```python
from build123d import *

# Parameters (mm, degrees)
BOSS_EXTRUDE2_DEPTH = 5
SKETCH2_R           = 2.5
CUT_EXTRUDE1_DEPTH  = 5
SKETCH3_R           = 7
SKETCH3_R_2         = 1
CUT_EXTRUDE2_DEPTH  = 90.644870735
SKETCH4_R           = 1.5
CUT_EXTRUDE3_DEPTH  = 90.644870735
SKETCH5_R           = 1
CUT_EXTRUDE4_DEPTH  = 90.644870735


with BuildPart() as part:
    # Sketch1 → Boss-Extrude2 (new body)
    with BuildSketch(Plane(origin=(0, 0, 0), x_dir=(-1, 0, 0), z_dir=(0, 1, 0))):
        Polygon((-72.491053579, -52.5), (42.508946421, -52.5), (28.132122167, -13), (-65.526137841, -13), align=None)
    extrude(amount=BOSS_EXTRUDE2_DEPTH)

    # Sketch2 → Cut-Extrude1 (cut)
    with BuildSketch(Plane(origin=(0, 5, 0), x_dir=(-1, 0, 0), z_dir=(0, 1, 0))):
        with Locations(Location((28.227466353, -42.5, 0), (0, 0, 90))):
            Circle(SKETCH2_R)
        with Locations(Location((0, -22.5, 0), (0, 0, 90))):
            Circle(SKETCH2_R)
        with Locations(Location((-60.573517653, -42.5, 0), (0, 0, 90))):
            Circle(SKETCH2_R)
    extrude(amount=-CUT_EXTRUDE1_DEPTH, mode=Mode.SUBTRACT)

    # Sketch3 → Cut-Extrude2 (cut, through all)
    with BuildSketch(Plane(origin=(0, 5, 0), x_dir=(1, 0, 0), z_dir=(0, 1, 0))):
        with Locations(Location((29.491053579, 32, 0), (0, 0, 270))):
            Circle(SKETCH3_R)
        with Locations(Location((20.491053579, 32, 0), (0, 0, 270))):
            Circle(SKETCH3_R_2)
        with Locations(Location((29.491053579, 41, 0), (0, 0, 270))):
            Circle(SKETCH3_R_2)
        with Locations(Location((38.491053579, 32, 0), (0, 0, 270))):
            Circle(SKETCH3_R_2)
        with Locations(Location((29.491053579, 23, 0), (0, 0, 270))):
            Circle(SKETCH3_R_2)
    extrude(amount=-CUT_EXTRUDE2_DEPTH, mode=Mode.SUBTRACT)

    # Sketch4 → Cut-Extrude3 (cut, through all)
    with BuildSketch(Plane.XZ):
        with Locations(Location((-24.785336663, -15.5, 0), (0, 0, 270))):
            Circle(SKETCH4_R)
        with Locations(Location((10.214663337, -15.5, 0), (0, 0, 270))):
            Circle(SKETCH4_R)
        with Locations(Location((45.214663337, -15.5, 0), (0, 0, 270))):
            Circle(SKETCH4_R)
        with Locations(Location((63.861406816, -17.95576741, 0), (0, 0, 270))):
            Circle(SKETCH4_R)
        with Locations(Location((66.466129481, -32.727883705, 0), (0, 0, 270))):
            Circle(SKETCH4_R)
        with Locations(Location((69.070852146, -47.5, 0), (0, 0, 270))):
            Circle(SKETCH4_R)
    extrude(amount=-CUT_EXTRUDE3_DEPTH, mode=Mode.SUBTRACT)

    # Sketch5 → Cut-Extrude4 (cut, through all)
    with BuildSketch(Plane(origin=(0, 5, 0), x_dir=(-1, 0, 0), z_dir=(0, 1, 0))):
        with Locations(Location((37.295727555, -46.948212084, 0), (0, 0, 90))):
            Circle(SKETCH5_R)
    extrude(amount=-CUT_EXTRUDE4_DEPTH, mode=Mode.SUBTRACT)


solid = part.part
```
Here's how the part is built. I have some questions about the finished solid (model axes, mm). Give positions to 0.01 mm unless a question says otherwise; leave off trailing zeros. Write each loop counter-clockwise with the first axis right and the second up, starting at its lowest first coordinate (ties: lowest second). Pieces come first, ordered by that corner, then holes. Notation, with made-up numbers: M 35.5,-17.5 L 53.5,-17.5 A25 cw 53.5,10.5 Z; hole C -5.5,14.5 d10. An arc over 180 degrees is marked long. Put each result on its own line as item: value. Start each with the question number.
Item 1: I need wall thicknesses on L1, parallel to Z at x = 29.5, y = 3.3; L2, parallel to Z at x = 10, y = 0.3; L3, parallel to X at y = 4.5, z = -16. Which ranges of each line are inside material? Lowest first, please. Write a range as from..to.
Item 2: If we section it at C-C, the plane y = 2.95: Count the separate pieces of the cut face and the enclosed holes in it, then the cut area to 3 significant figures.
Item 3: Thinking about a two-plate mould opening in Z: for faces 1 (the flat face through (16, 0, -32)), 2 (the cylindrical face through (68.16, 2.46, -46.31)), 3 (the flat face through (16, 2, -52.5)), which applies, +Z half, -Z half, draft (parallel to the pull), parting line (faces both ways), or undercut?
Item 4: Will this pin go through, and if not, where does the flat tip stop? pin 1 (8.5 mm diameter, centred on x = 29.49, z = -32, fed in from -Y).
Item 5: If we section it at A-A, the plane z = -38: Write out the boundary of the cut face in (x, y), then the cut area to 3 significant figures.
Item 6: If we section it at B-B, the plane z = -23: Write out the boundary of the cut face in (x, y), then the cut area to 3 significant figures.
Values:
1. L1: -52.5..-42, -40..-39, -25..-24, -22..-13
1. L2: -52.5..-16.98, -14.02..-13
1. L3: -29.22..-26.2, -23.37..8.8, 11.63..43.8, 46.63..66.06
2. separate pieces: 1
2. enclosed holes: 15
2. area: 3,850 mm²
3. face 1: draft
3. face 2: undercut
3. face 3: -Z half
4. pin 1: through
5. outline: M -37.23,0 L 25.89,0 L 25.89,5 L -37.23,5 Z; M 33.1,0 L 69.93,0 L 69.93,5 L 33.1,5 Z
5. area: 500 mm²
6. outline: M -31.77,0 L -2.45,0 L -2.45,5 L -31.77,5 Z; M 2.45,0 L 28.49,0 L 28.49,5 L 2.45,5 Z; M 30.49,0 L 67.29,0 L 67.29,5 L 30.49,5 Z
6. area: 461 mm²
